Work out the finished part from the listing and answer in its coordinate system (mm). A direction names the side the tool comes from. Coordinates: 2 decimals unless noted, no trailing zeros. Loops run counter-clockwise (first coordinate to the right, second up) from the corner with the lowest first, then second, coordinate; pieces in that order, holes last. Notation, with made-up numbers: (-14, 75) -> (-3, 75) arc R25 cw to (-3, 97) -> close; hole circle Ø11 at (64, -5). An arc over 180 degrees is marked (long way). Use a Markdown table: item, result.
from build123d import *

# Parameters (mm, degrees)
EXTRUDE_1_DEPTH = 1000


with BuildPart() as part:
    # Эскиз1 → Бобышка-Вытянуть1 (new body)
    with BuildSketch(Plane.XY):
        with BuildLine():
            Line((0, 38.5), (0, 1.5))
            ThreePointArc((0, 1.5), (0.439339828, 0.439339828), (1.5, 0))
            Line((1.5, 0), (18.5, 0))
            ThreePointArc((18.5, 0), (19.560660172, 0.439339828), (20, 1.5))
            Line((20, 1.5), (20, 38.5))
            ThreePointArc((20, 38.5), (19.560660172, 39.560660172), (18.5, 40))
            Line((18.5, 40), (1.5, 40))
            ThreePointArc((1.5, 40), (0.439339828, 39.560660172), (0, 38.5))
        make_face()
        with BuildLine():
            Line((1.5, 37.5), (1.5, 2.5))
            ThreePointArc((1.5, 2.5), (1.792893219, 1.792893219), (2.5, 1.5))
            Line((2.5, 1.5), (17.5, 1.5))
            ThreePointArc((17.5, 1.5), (18.207106781, 1.792893219), (18.5, 2.5))
            Line((18.5, 2.5), (18.5, 37.5))
            ThreePointArc((18.5, 37.5), (18.207106781, 38.207106781), (17.5, 38.5))
            Line((17.5, 38.5), (2.5, 38.5))
            ThreePointArc((2.5, 38.5), (1.792893219, 38.207106781), (1.5, 37.5))
        make_face(mode=Mode.SUBTRACT)
    extrude_1 = extrude(amount=EXTRUDE_1_DEPTH)

    # Зеркальное отражение1: Бобышка-Вытянуть1 across plane
    add(extrude_1.mirror(Plane(origin=(18.5, 38.5, 0), x_dir=(1, 0, 0), z_dir=(0, 0, -1))))


solid = part.part
Q1. Consider line 1 (Y direction, x = 7.25, z = -484.5); line 2 (Y direction, x = 18, z = 834.5); line 3 (X direction, y = 16, z = -171). Determine where each line is inside the solid, lowest interval first. Write a range as [from, to].
Solved:
| item | result |
|---|---|
| line 1 | [0, 1.5], [38.5, 40] |
| line 2 | [0, 1.63], [38.37, 40] |
| line 3 | [0, 1.5], [18.5, 20] |
Q2. Section B-B on y = 20 is taken. Determine the outline of the cut face in (x, z).
Solved:
| item | result |
|---|---|
| outline | (0, -1000) -> (1.5, -1000) -> (1.5, 1000) -> (0, 1000) -> close; (18.5, -1000) -> (20, -1000) -> (20, 1000) -> (18.5, 1000) -> close |
Q3. Section C-C on z = 835 is taken. Determine the outline of the cut face in (x, y), and give its area (3 significant figures).
Solved:
| item | result |
|---|---|
| outline | (0, 1.5) arc R1.5 ccw to (1.5, 0) -> (18.5, 0) arc R1.5 ccw to (20, 1.5) -> (20, 38.5) arc R1.5 ccw to (18.5, 40) -> (1.5, 40) arc R1.5 ccw to (0, 38.5) -> close; hole (1.5, 2.5) arc R1 ccw to (2.5, 1.5) -> (17.5, 1.5) arc R1 ccw to (18.5, 2.5) -> (18.5, 37.5) arc R1 ccw to (17.5, 38.5) -> (2.5, 38.5) arc R1 ccw to (1.5, 37.5) -> close |
| area | 170 mm² |
Q4. For faces 1 (the flat face through (1.5, 20, 14)), 2 (the flat face through (20, 20, 14)), determine the directions among +Z, -Z, +X, -X, +Y, -Y from which every point of the face is accessible in a straight line to the end or side of a thin tool.
Solved:
| item | result |
|---|---|
| face 1 | +Z, -Z |
| face 2 | +Z, -Z, +X, +Y, -Y |
Q5. Section A-A on x = 13.5 is taken. Determine the outline of the cut face in (y, z), and give its area (3 significant figures).
Solved:
| item | result |
|---|---|
| outline | (0, -1000) -> (1.5, -1000) -> (1.5, 1000) -> (0, 1000) -> close; (38.5, -1000) -> (40, -1000) -> (40, 1000) -> (38.5, 1000) -> close |
| area | 6,000 mm² |
